Input: part model. Units: mm. Frame: model coordinates. A direction names the side the tool comes from. Round coordinates to 2 decimals unless told otherwise and drop trailing zeros. Loops run counter-clockwise (first coordinate to the right, second up) from the corner with the lowest first, then second, coordinate; pieces in that order, holes last.
1) First-contact query: pin 1 (1.7 mm diameter, centred on y = -1.5, z = -16.5, fed in from +X); pin 2 (1.1 mm diameter, centred on x = -7.5, z = -0.5, fed in from -Y); pin 3 (1.1 mm diameter, centred on x = 4.5, y = -1.5, fed in from -Z). Flat tips, straight axial feed; report the tip coordinate or a pass-through.
2) Access query for faces 4 (the face through (-2.9, -1.6, -4.234)), 5 (the face through (5, -1, -15.3)), 6 (the face through (5, -1, 15.3)). Directions: +Z, -Z, +X, -X, +Y, -Y. A direction counts if a zero-diameter tool reaches every point of the face in a straight line with its end or side. Return the directions, or none.
3) Section D-D, the plane z = 1. Return loops of the section in (x, y).
4) Section A-A, the plane y = -0.65. Return loops of the section in (x, z).
5) Section C-C, the plane z = -11. Return loops of the section in (x, y).
6) Draft query along X for faces 1 (the face through (10.5, -1, -12)), 2 (the face through (-10.49, -1, 14)), 3 (the face through (3.83, -2.086, 7.007)). Return one class per face: pulls with the +X half, pulls with the -X half, needs draft (parallel to the pull), parting line crosses it, or undercut.
7) Section B-B, the plane x = -5. Return loops of the section in (y, z), and give its area (3 significant figures).
8) Ray query, line 1 along X through (y, z) = (-1.6, 6.5); line 2 along Y through (x, z) = (1, -11); line 3 along X through (y, z) = (-0.55, -11). Return the intervals inside material, ascending.
from build123d import *

# Parameters (mm, degrees)
F1_DEPTH = 2.1
F2_R     = 1.955848
F2_R_2   = 0.950029
F3_DEPTH = 1.016
F2_R_3   = 2.811265
F2_R_4   = 1.91782
F4_DEPTH = 1.016


with BuildPart() as f1:
    # F0 (on Front) → F1 (new body)
    with BuildSketch(Plane.XZ):
        with BuildLine():
            Line((-10.4902, 18.4), (-10.4902, 9.27123))
            ThreePointArc((-10.4902, 9.27123), (-14, 0), (-10.4902, -9.27123))
            Line((-10.4902, -9.27123), (-10.4902, -18.4))
            Line((-10.4902, -18.4), (0, -18.4))
            Line((0, -18.4), (0, -15.3))
            Line((0, -15.3), (10.5, -15.3))
            Line((10.5, -15.3), (10.5, -9.26013))
            ThreePointArc((10.5, -9.26013), (14, 0), (10.5, 9.26013))
            Line((10.5, 9.26013), (10.5, 15.3))
            Line((10.5, 15.3), (0, 15.3))
            Line((0, 15.3), (0, 18.4))
            Line((0, 18.4), (-10.4902, 18.4))
        make_face()
    extrude(amount=F1_DEPTH)

    # F2 (on face) → F3 (cut)
    with BuildSketch(Plane.XZ.offset(2.1)):
        Polygon((-5.717198, -4.234256), (-7.893182, 2.19699), (-7.893182, -4.234256), align=None)
        Polygon((-4.314896, 2.19699), (-6.249105, 2.19699), (-3.928055, -4.234256), (-1.897135, -4.234256), align=None)
        Polygon((-1.075096, 2.19699), (-2.574108, 2.19699), (0, -4.234256), (1.777862, -4.234256), align=None)
        Polygon((2.019639, 2.19699), (0.472271, 2.19699), (3.567006, -4.234256), (5.307794, -4.234256), align=None)
        Polygon((5.211083, 2.19699), (3.567006, 2.19699), (6.419964, -4.234256), (7.628845, -4.234256), align=None)
        Polygon((8.837725, 2.19699), (6.419963, 2.19699), (8.837725, -4.234256), align=None)
        with Locations((-5.330356, 6.065408)):
            Circle(F2_R)
        with Locations((3.953848, 6.065408)):
            Circle(F2_R_2)
    extrude(amount=-F3_DEPTH, mode=Mode.SUBTRACT)

    # F2 (on face) → F4 (join)
    with BuildSketch(Plane.XZ.offset(2.1)):
        with Locations((-5.330356, 6.065408)):
            Circle(F2_R_3)
        with Locations((-5.330356, 6.065408)):
            Circle(F2_R, mode=Mode.SUBTRACT)
        with Locations((3.953848, 6.065408)):
            Circle(F2_R_4)
        with Locations((3.953848, 6.065408)):
            Circle(F2_R_2, mode=Mode.SUBTRACT)
    extrude(amount=F4_DEPTH)


solid = f1.part
Final values:
1. pin 1: stops at x = 0
1. pin 2: stops at y = -2.1
1. pin 3: stops at z = -15.3
2. face 4: -Y
2. face 5: -Z, +X, +Y, -Y
2. face 6: +Z, +X, +Y, -Y
3. outline: (-13.96, -2.1) - (-7.89, -2.1) - (-7.89, -1.08) - (-7.49, -1.08) - (-7.49, -2.1) - (-5.82, -2.1) - (-5.82, -1.08) - (-3.86, -1.08) - (-3.86, -2.1) - (-2.1, -2.1) - (-2.1, -1.08) - (-0.54, -1.08) - (-0.54, -2.1) - (1.05, -2.1) - (1.05, -1.08) - (2.63, -1.08) - (2.63, -2.1) - (4.1, -2.1) - (4.1, -1.08) - (5.66, -1.08) - (5.66, -2.1) - (6.87, -2.1) - (6.87, -1.08) - (8.84, -1.08) - (8.84, -2.1) - (13.96, -2.1) - (13.96, 0) - (-13.96, 0) - close
4. outline: (-10.49, -18.4) - (0, -18.4) - (0, -15.3) - (10.5, -15.3) - (10.5, -9.26) arc R14 ccw to (10.5, 9.26) - (10.5, 15.3) - (0, 15.3) - (0, 18.4) - (-10.49, 18.4) - (-10.49, 9.27) arc R14 ccw to (-10.49, -9.27) - close
5. outline: (-10.49, -2.1) - (10.5, -2.1) - (10.5, 0) - (-10.49, 0) - close
6. face 1: pulls with the +X half
6. face 2: pulls with the -X half
6. face 3: undercut
7. outline: (-3.12, 3.27) - (-2.1, 3.27) - (-2.1, 2.2) - (-1.08, 2.2) - (-1.08, -1.26) - (-2.1, -1.26) - (-2.1, -18.4) - (0, -18.4) - (0, 18.4) - (-2.1, 18.4) - (-2.1, 8.86) - (-3.12, 8.86) - (-3.12, 7.99) - (-1.08, 7.99) - (-1.08, 4.14) - (-3.12, 4.14) - close
7. area: 71.6 mm2
8. line 1: x = -12.4 to -7.24, -3.42 to 3.11, 4.8 to 12.4
8. line 2: y = -2.1 to 0
8. line 3: x = -10.49 to 10.5
